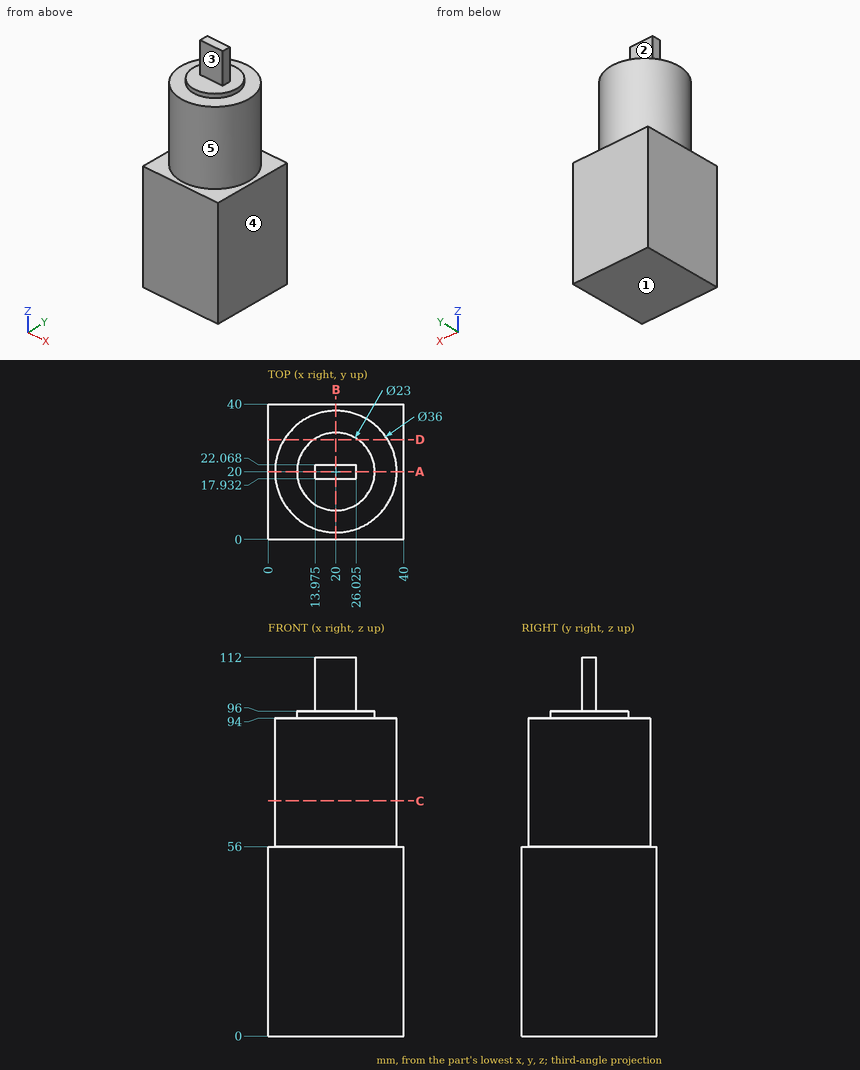
For this review, use the dimensioned drawing (mm, ordinates from the lowest corner) and the shaded views. A direction names the side the tool comes from. Round coordinates to 2 decimals unless told otherwise and drop trailing zeros. Write each loop counter-clockwise with the first axis right and the second up, starting at its lowest first coordinate (ties: lowest second). Pieces come first, ordered by that corner, then holes. Notation, with made-up numbers: (-16.5, -28.5) - (30.5, -28.5) arc R16 cw to (30.5, -15.5) - close; hole circle Ø8 at (-10, 26.5). An arc over 180 degrees is marked (long way). Answer as a JSON object with one key per item and string values.
1. We need section D-D on y = 29.5. Give the boundary of the cut face in (x, z), then the cut area to 3 significant figures.
Response values:
{"outline": "(0, 0) - (40, 0) - (40, 56) - (35.29, 56) - (35.29, 94) - (26.48, 94) - (26.48, 96) - (13.52, 96) - (13.52, 94) - (4.71, 94) - (4.71, 56) - (0, 56) - close", "area": "3,430 mm2"}
2. We need section B-B on x = 20. Give the boundary of the cut face in (y, z).
Response values:
{"outline": "(0, 0) - (40, 0) - (40, 56) - (38, 56) - (38, 94) - (31.5, 94) - (31.5, 96) - (22.07, 96) - (22.07, 112) - (17.93, 112) - (17.93, 96) - (8.5, 96) - (8.5, 94) - (2, 94) - (2, 56) - (0, 56) - close"}
3. We need section A-A on y = 20. Give the boundary of the cut face in (x, z) (1 decimal), then the cut area to 3 significant figures.
Response values:
{"outline": "(0, 0) - (40, 0) - (40, 56) - (38, 56) - (38, 94) - (31.5, 94) - (31.5, 96) - (26, 96) - (26, 112) - (14, 112) - (14, 96) - (8.5, 96) - (8.5, 94) - (2, 94) - (2, 56) - (0, 56) - close", "area": "3,850 mm2"}
4. Tool access review of the marked faces 1, 2, 3, 4 and 5: name each direction out of +Z, -Z, +X, -X, +Y, -Y from which nothing blocks a thin tool from reaching the whole face with its end or side.
Response values:
{"face 1": "-Z, +X, -X, +Y, -Y", "face 2": "+Z, +X, -X, +Y", "face 3": "+Z, +X, -X, -Y", "face 4": "+Z, -Z, +X, +Y, -Y", "face 5": "+Z"}
5. For pin 1 Ø10 at (y, z) = (27, 84.5) entering from +X; pin 2 Ø1 at (y, z) = (19.5, 57) entering from -X; pin 3 Ø8 at (y, z) = (34.5, 73.5) entering from -X, all flat-tipped, find the tip position at first contact; note any pin that passes through.
Response values:
{"pin 1": "stops at x = 37.89", "pin 2": "stops at x = 2", "pin 3": "stops at x = 5.38"}
6. We need section C-C on z = 69.5. Give the boundary of the cut face in (x, y).
Response values:
{"outline": "circle Ø36 at (20, 20)"}
7. To check wall thickness, follow line 1 along Y through (x, z) = (25, 101.5); line 2 along Z through (x, y) = (7.5, 9); line 3 along X through (y, z) = (19.5, 100) (1 decimal). State the ranges of each line that lie inside material, in increasing order.
Response values:
{"line 1": "y = 17.93 to 22.07", "line 2": "z = 0 to 94", "line 3": "x = 14 to 26"}
